The listing builds one solid part. Answer for the finished solid, in the listing's coordinates (mm). A direction names the side the tool comes from. Coordinates: 2 decimals unless noted, no trailing zeros. Order: outer loops, then holes, each group sorted by start corner. A loop starts at its lowest first (then second) coordinate and runs counter-clockwise, first axis right, second up. Notation, with made-up numbers: (77, -17.5) -> (93, -17.5) arc R23 cw to (93, 19.5) -> close; hole circle Ø1 at (-1.75, 60.5). An arc over 180 degrees is marked (long way). Return JSON: item names as keys, results as strings.
from build123d import *

# Parameters (mm, degrees)
BOSS_EXTRUDE1_DEPTH                                  = 22.05
BOSS_EXTRUDE1_DEPTH_BACK                             = 5.45
BOSS_EXTRUDE1_2_DEPTH                                = 22.05
BOSS_EXTRUDE1_2_DEPTH_BACK                           = 5.45
SKETCH3_W                                            = 51.63175717
SKETCH3_H                                            = 2.803707317
CUT_EXTRUDE1_DEPTH                                   = 4.5
SKETCH5_W                                            = 5
SKETCH5_H                                            = 4.5
BOSS_EXTRUDE2_DEPTH                                  = 0.35
SKETCH4_W                                            = 3.5
SKETCH4_H                                            = 1
CUT_EXTRUDE2_DEPTH                                   = 3.5
BOSS_EXTRUDE3_DEPTH                                  = 16.05
SHELL3_START                                         = -16.05
SHELL3_OUTLINE_R                                     = 26.3
SHELL3_DEPTH                                         = 13.35
F_2_0_2_DIAMETER_HOLE1_D                             = 2
CSK_SLOT_FOR_M2_COUNTERSUNK_FLAT_HEAD_SC_D           = 2.4
CSK_SLOT_FOR_M2_COUNTERSUNK_FLAT_HEAD_SC_CSINK_D     = 4.4
CSK_SLOT_FOR_M2_COUNTERSUNK_FLAT_HEAD_SC_CSINK_ANGLE = 90


# Read off the part's stored shape, not the designer's step: Shell3
with BuildPart() as part:
    # Sketch2 → Boss-Extrude1 (new, two sides: drawn at the far end of the back side and taken through both)
    with BuildSketch(Plane.XY.offset(-BOSS_EXTRUDE1_DEPTH_BACK)):
        Polygon((-11.25, 0), (-11.25, 2.6), (-12.5, 2.6), (-12.5, 5.1), (-7.5, 5.1), (-7.5, 2.6), (-8.75, 2.6), (-8.75, 0), align=None)
    extrude(amount=BOSS_EXTRUDE1_DEPTH + BOSS_EXTRUDE1_DEPTH_BACK)


with BuildPart() as body_2:
    # Sketch2 → Boss-Extrude1 2 (new, two sides: drawn at the far end of the back side and taken through both)
    with BuildSketch(Plane.XY.offset(-BOSS_EXTRUDE1_2_DEPTH_BACK)):
        Polygon((8.75, 0), (11.25, 0), (11.25, 2.6), (12.5, 2.6), (12.5, 5.1), (7.5, 5.1), (7.5, 2.6), (8.75, 2.6), align=None)
    extrude(amount=BOSS_EXTRUDE1_2_DEPTH + BOSS_EXTRUDE1_2_DEPTH_BACK)


with BuildPart() as cut_extrude1_tool:
    # Sketch3 → Cut-Extrude1 (new body)
    with BuildSketch(Plane(origin=(0, 0, -5.45), x_dir=(-1, 0, 0), z_dir=(0, 0, -1))):
        with Locations((1.197864232, 3.698146342)):
            Rectangle(SKETCH3_W, SKETCH3_H)
    extrude(amount=-CUT_EXTRUDE1_DEPTH)


with BuildPart() as part_1:
    add(part.part)

    # Cut-Extrude1: cut by cut_extrude1_tool
    add(cut_extrude1_tool.part, mode=Mode.SUBTRACT)



with BuildPart() as body_2_1:
    add(body_2.part)

    # Cut-Extrude1: cut by cut_extrude1_tool
    add(cut_extrude1_tool.part, mode=Mode.SUBTRACT)


with BuildPart() as part_2:
    add(part_1.part)

    add(body_2_1.part)  # Boss-Extrude2 merges body 2
    # Sketch5 → Boss-Extrude2 (add)
    with BuildSketch(Plane(origin=(0, 2.296292683, 0), x_dir=(1, 0, 0), z_dir=(0, 1, 0))):
        with Locations((10, 3.2)):
            Rectangle(SKETCH5_W, SKETCH5_H)
        with Locations((-10, 3.2)):
            Rectangle(SKETCH5_W, SKETCH5_H)
    extrude(amount=BOSS_EXTRUDE2_DEPTH)

    # Sketch4 → Cut-Extrude2 (cut)
    with BuildSketch(Plane(origin=(0, 0, -0.95), x_dir=(-1, 0, 0), z_dir=(0, 0, -1))):
        with Locations((10, 3.85)):
            Rectangle(SKETCH4_W, SKETCH4_H)
        with Locations((-10, 3.85)):
            Rectangle(SKETCH4_W, SKETCH4_H)
    extrude(amount=-CUT_EXTRUDE2_DEPTH, mode=Mode.SUBTRACT)

    # Sketch1 → Boss-Extrude3 (add)
    with BuildSketch(Plane(origin=(0, 0, 0), x_dir=(1, 0, 0), z_dir=(0, 1, 0))):
        with BuildLine():
            ThreePointArc((-29, -7.4e-08), (-26.336723438, -12.139892855), (-18.836069123, -22.05))
            Line((-18.836069123, -22.05), (18.836069123, -22.05))
            ThreePointArc((18.836069123, -22.05), (26.336723454, -12.139892822), (29, 0))
            ThreePointArc((29, 0), (-3.7e-08, 29), (-29, -7.4e-08))
        make_face()
        with BuildLine():
            Line((18.836069123, -22.05), (-18.836069123, -22.05))
            ThreePointArc((-18.836069123, -22.05), (0, -29), (18.836069123, -22.05))
        make_face()
    extrude(amount=-BOSS_EXTRUDE3_DEPTH)

    # Shell3 outline → Shell3 (cut)
    with BuildSketch(Plane(origin=(0, 0, 0), x_dir=(1, 0, 0), z_dir=(0, 1, 0)).offset(SHELL3_START)):
        Circle(SHELL3_OUTLINE_R)
    extrude(amount=SHELL3_DEPTH, mode=Mode.SUBTRACT)

    # Ø2.0 (2) Diameter Hole1 (through all)
    with Locations(Plane(origin=(0, 5.1, 0), x_dir=(1, 0, 0), z_dir=(0, 1, 0))):
        with Locations((10, -2.6), (-10, -2.6)):
            Hole(F_2_0_2_DIAMETER_HOLE1_D / 2)

    # CSK SLOT for M2 Countersunk Flat Head Screw3 (through all)
    with Locations(Plane(origin=(0, 0, 0), x_dir=(1, 0, 0), z_dir=(0, 1, 0))):
        with Locations((-16.001826458, -16.001826458), (16.001826458, 16.001826458)):
            CounterSinkHole(CSK_SLOT_FOR_M2_COUNTERSUNK_FLAT_HEAD_SC_D / 2, CSK_SLOT_FOR_M2_COUNTERSUNK_FLAT_HEAD_SC_CSINK_D / 2, counter_sink_angle=CSK_SLOT_FOR_M2_COUNTERSUNK_FLAT_HEAD_SC_CSINK_ANGLE)


solid = part_2.part
1. The part is cut by section A-A on x = 0. Give the vertices of the cut face in (y, z), and give its area (3 significant figures).
Answer block:
{"outline": "(-16.05, -29) -> (0, -29) -> (0, 29) -> (-16.05, 29) -> (-16.05, 26.3) -> (-2.7, 26.3) -> (-2.7, -26.3) -> (-16.05, -26.3) -> close", "area": "229 mm2"}
2. For faces 1 (the face through (-10, 2.646, -3)), 2 (the face through (-12.5, 4, 8)), 3 (the face through (12.5, 4, 8)), 4 (the face through (7.5, 4, 8)), 5 (the face through (-10, 3.35, 1)), determine the directions among +Z, -Z, +X, -X, +Y, -Y from which every point of the face is accessible in a straight line to the end or side of a thin tool.
Answer block:
{"face 1": "-Z, +X, -X, +Y", "face 2": "+Z, -Z, -X, +Y", "face 3": "+Z, -Z, +X, +Y", "face 4": "+Z, -Z, +Y", "face 5": "-Z"}
3. The part is cut by section C-C on z = -9. Give the vertices of the cut face in (x, y), and give its area (3 significant figures).
Answer block:
{"outline": "(-27.57, -16.05) -> (-24.71, -16.05) -> (-24.71, -2.7) -> (24.71, -2.7) -> (24.71, -16.05) -> (27.57, -16.05) -> (27.57, 0) -> (-27.57, 0) -> close", "area": "225 mm2"}
4. Consider line 1 (Z direction, x = -10, y = 1.25); line 2 (Y direction, x = -12, z = -3); line 3 (Y direction, x = 24, z = -10). Determine where each line is inside the solid, lowest interval first. Write a range as from..to.
Answer block:
{"line 1": "z = -5.45..1.6, 3.6..22.05", "line 2": "y = -2.7..0, 2.3..2.65", "line 3": "y = -2.7..0"}
5. Each of these flat-tipped pins is pushed along its axis until it touches: pin 1 Ø4 at (x, z) = (-16, 16) entering from +Y; pin 2 Ø0.8 at (y, z) = (4.5, 10) entering from -X; pin 3 Ø1.5 at (y, z) = (-3, 11.5) entering from -X; pin 4 Ø8 at (y, z) = (-1, -2.5) entering from +X. Where does it stop, or does it pass through?
Answer block:
{"pin 1": "stops at y = -0.2", "pin 2": "stops at x = -12.5", "pin 3": "stops at x = -26.93", "pin 4": "stops at x = 29"}
6. Determine the mould class of faces 6 (the face through (10, 5.1, 10)), 7 (the face through (10.217, 1.145, 3.576)), 8 (the face through (10, 3, -0.95)) for opening direction Z: pulls with the +Z half, pulls with the -Z half, needs draft (parallel to the pull), parting line crosses it, or undercut.
Answer block:
{"face 6": "needs draft", "face 7": "undercut", "face 8": "pulls with the -Z half"}
7. The part is cut by section B-B on y = -11. Give the vertices of the cut face in (x, z).
Answer block:
{"outline": "circle Ø58 at (0, 0); hole circle Ø52.6 at (0, 0)"}
8. The part is cut by section D-D on x = 10. Give the vertices of the cut face in (y, z), and give its area (3 significant figures).
Answer block:
{"outline": "(-16.05, -27.22) -> (0, -27.22) -> (0, -5.45) -> (2.65, -5.45) -> (2.65, -0.95) -> (3.35, -0.95) -> (3.35, 1.6) -> (-2.7, 1.6) -> (-2.7, -24.32) -> (-16.05, -24.32) -> close; (-16.05, 24.32) -> (-2.7, 24.32) -> (-2.7, 3.6) -> (5.1, 3.6) -> (5.1, 22.05) -> (0, 22.05) -> (0, 27.22) -> (-16.05, 27.22) -> close; (4.35, -0.95) -> (5.1, -0.95) -> (5.1, 1.6) -> (4.35, 1.6) -> close", "area": "335 mm2"}
